Can you work these out from the drawing? Everything is in mm from the part's minimum corner. A direction names the side the tool comes from. Give positions to 0.01 mm unless a question says otherwise; leave off trailing zeros. Write each loop counter-clockwise with the first axis right and the second up, starting at its lowest first coordinate (ties: lowest second). Pieces come first, ordered by that corner, then holes. Notation, with made-up numbers: (-21, 15.25) -> (-16, 15.25) arc R12 ccw to (-16, 32.25) -> close; hole circle Ø3 at (74, 2). An arc over 180 degrees is marked (long way). Use one line per item in the form item = value.
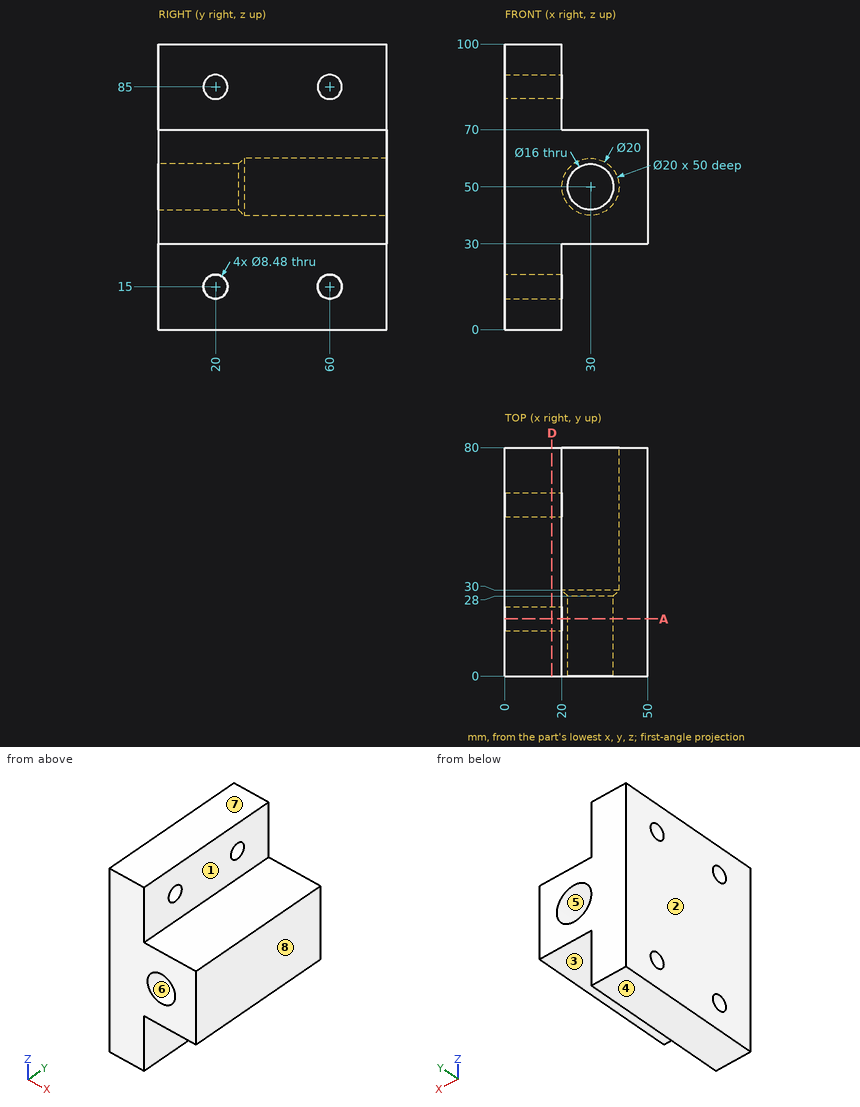
Q1. Which directions (+Z, -Z, +X, -X, +Y, -Y) give clear straight access to the entire face, cutting with the end or side of a thin tool? Please do the marked faces 1, 2, 3, 4 and 5.
Result set:
face_1 = +Z, +X, +Y, -Y
face_2 = +Z, -Z, -X, +Y, -Y
face_3 = -Z, +X, +Y, -Y
face_4 = -Z, +X, -X, +Y, -Y
face_5 = +Y
Q2. I want a section at A-A, the plane y = 20. Write out the boundary of the cut face in (x, z).
Result set:
outline = (0, 0) -> (20, 0) -> (20, 10.76) -> (0, 10.76) -> close; (0, 19.24) -> (20, 19.24) -> (20, 30) -> (50, 30) -> (50, 70) -> (20, 70) -> (20, 80.76) -> (0, 80.76) -> close; (0, 89.24) -> (20, 89.24) -> (20, 100) -> (0, 100) -> close; hole circle Ø16 at (30, 50)
Q3. Will these pins go through, and if not, where does the flat tip stop? pin 1 Ø1.5 at (y, z) = (37, 77) entering from -X; pin 2 Ø10 at (y, z) = (69.5, 21) entering from +X; pin 3 Ø9 at (x, y) = (42, 38.5) entering from +Z; pin 4 Ø10 at (x, y) = (26, 23) entering from -Z.
Result set:
pin_1 = 0
pin_2 = 20
pin_3 = 70
pin_4 = 30
Q4. If I drill on line 1 along Y through (x, z) = (10, 15); line 2 along X through (y, z) = (48, 50); line 3 along Y through (x, z) = (19.5, 82.5) (1 decimal), over which ranges is the centre line in solid material (lowest first)? Write a range as from..to.
Result set:
line_1 = 0..15.76, 24.24..55.76, 64.24..80
line_2 = 0..20, 40..50
line_3 = 0..16.6, 23.4..56.6, 63.4..80
Q5. If we mould it in two halves opening along X, with no side actions, what happens to the marked faces 6, 7 and 8? For each: +X half, -X half, draft (parallel to the pull), parting line (faces both ways), or undercut.
Result set:
face_6 = undercut
face_7 = draft
face_8 = +X half
Q6. I want a section at D-D, the plane x = 16.5. Write out the boundary of the cut face in (y, z), and give its area (3 significant figures).
Result set:
outline = (0, 0) -> (80, 0) -> (80, 100) -> (0, 100) -> close; hole circle Ø8.48 at (20, 15); hole circle Ø8.48 at (20, 85); hole circle Ø8.48 at (60, 15); hole circle Ø8.48 at (60, 85)
area = 7,770 mm2
